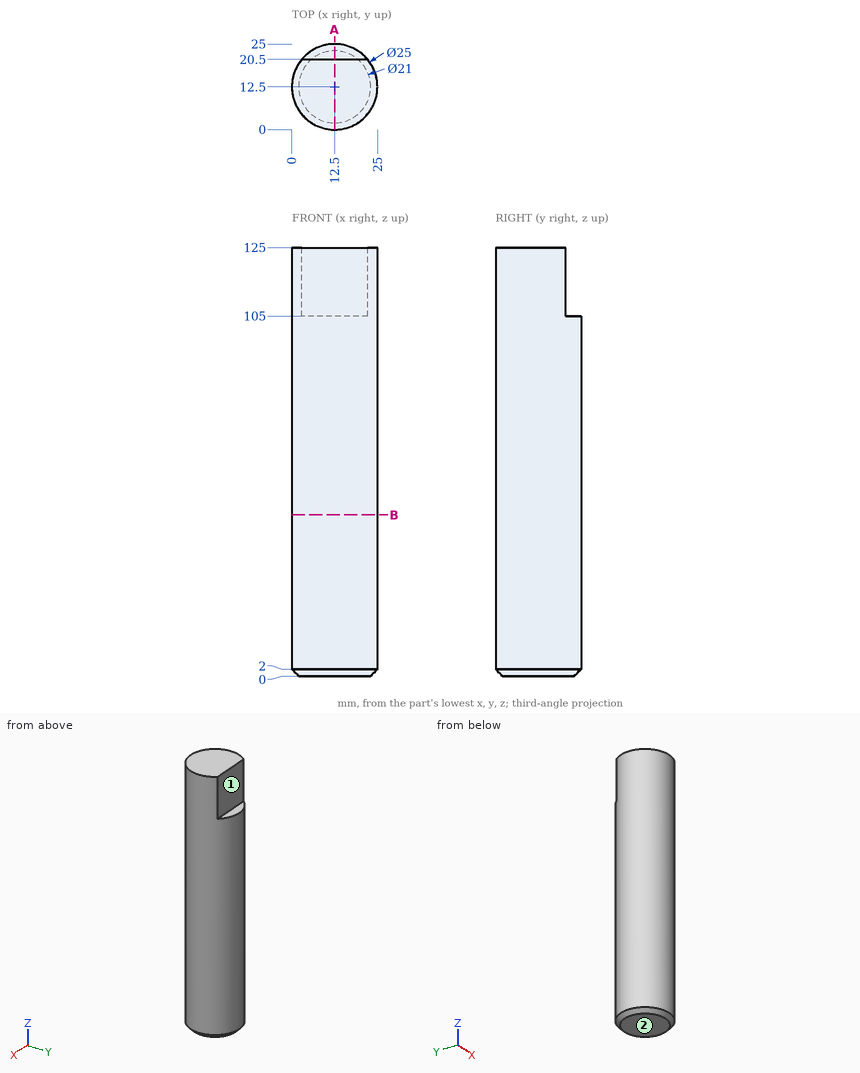
Job drawing, mm, ordinate dimensions from the low corner. One solid piece. A direction names the side the tool comes from. Coordinates: 2 decimals unless noted, no trailing zeros. Write each loop counter-clockwise with the first axis right and the second up, starting at its lowest first coordinate (ties: lowest second). Pieces come first, ordered by that corner, then holes. Notation, with made-up numbers: M 4,63 L 60,63 A12 cw 60,82 Z; hole C 39.5,12 d7. An arc over 180 degrees is marked long. Answer as a JSON object with one key per item and string values. Group by question number.
1) Pin check, flat tips, straight feed: pin 1 Ø5 at (y, z) = (20, 78) entering from +X; pin 2 Ø1.3 at (x, y) = (13, 23.5) entering from +Z; pin 3 Ø6 at (x, z) = (8, 17) entering from +Y. Stop position of each tip, or through.
2) Wall check: line 1 (Y direction, x = 5.75, z = 115); line 2 (Y direction, x = 13, z = 97); line 3 (X direction, y = 12.75, z = 112). Give the ranges that are in metal, low to high. Write a range as from..to.
3) Tool access for the marked faces 1 and 2: list every direction of +Z, -Z, +X, -X, +Y, -Y with a clear straight run to the whole face (end or side of a thin tool).
4) Saw through at A-A (x = 12.5). Write the cut outline in (y, z), plus the area to 3 significant figures.
5) Saw through at B-B (z = 47). Write the cut outline in (x, y).
Values follow:
{
 "1": {"pin 1": "stops at x = 23.96", "pin 2": "stops at z = 105", "pin 3": "stops at y = 24.91"},
 "2": {"line 1": "y = 1.98..20.5", "line 2": "y = 0.01..24.99", "line 3": "x = 0..25"},
 "3": {"face 1": "+Z, +X, -X, +Y", "face 2": "-Z, +X, -X, +Y, -Y"},
 "4": {"outline": "M 0,2 L 2,0 L 23,0 L 25,2 L 25,105 L 20.5,105 L 20.5,125 L 0,125 Z", "area": "3,030 mm2"},
 "5": {"outline": "C 12.5,12.5 d25"}
}
